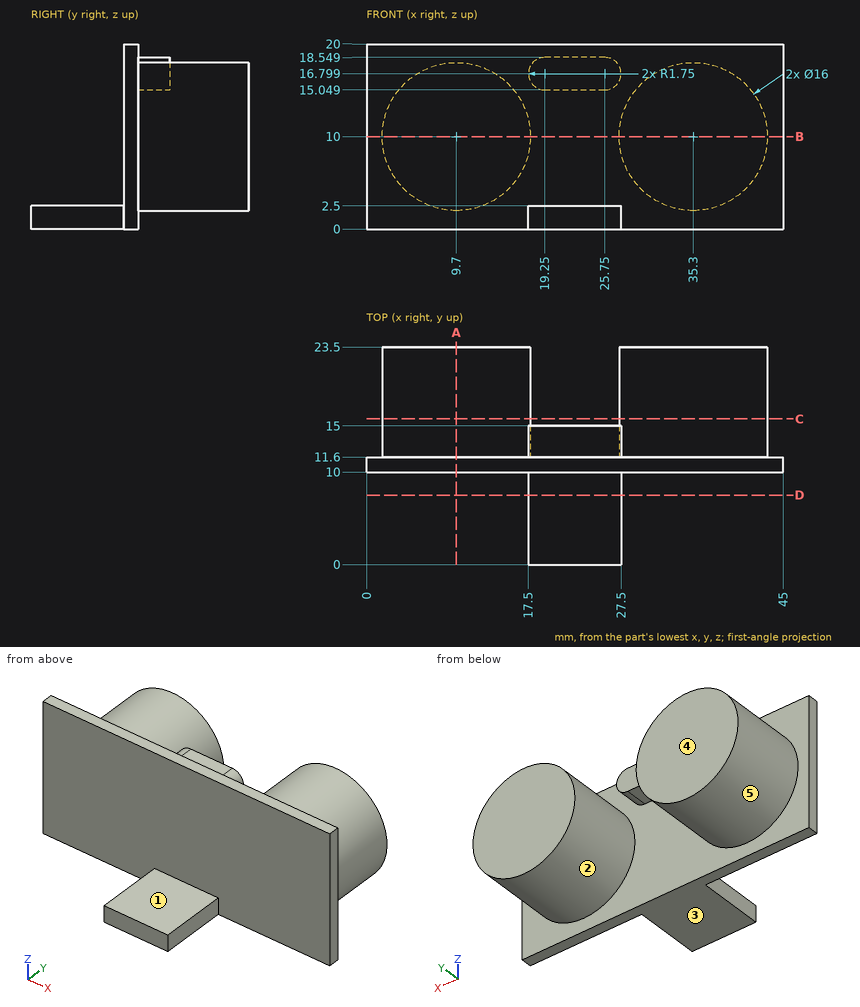
Can you work these out from the drawing? Everything is in mm from the part's minimum corner. A direction names the side the tool comes from. Round coordinates to 2 decimals unless told otherwise and drop trailing zeros. Loops run counter-clockwise (first coordinate to the right, second up) from the corner with the lowest first, then second, coordinate; pieces in that order, holes last. Notation, with made-up numbers: (-12, 2) - (-8, 2) arc R15 ccw to (-8, 25) - close; hole circle Ø1 at (-3, 57). An arc over 180 degrees is marked (long way). One line per question, with ' | ' between items. Start each with the question number.
Q1. I want a section at A-A (x = 9.7). Write out the boundary of the cut face in (y, z), then the cut area to 3 significant figures.
Q2. I want a section at B-B (z = 10). Write out the boundary of the cut face in (x, y).
Q3. I want a section at D-D (y = 7.5). Write out the boundary of the cut face in (x, z).
Q4. We'd pull the mould along X, two halves only. Please class the marked faces 4 and 5: +X half, -X half, draft (parallel to the pull), parting line (faces both ways), or undercut.
Q5. For the marked faces 1, 2 and 3, which set-ups out of +Z, -Z, +X, -X, +Y, -Y let a thin tool reach every point of the face, with its end or its side?
Q6. I want a section at C-C (y = 15.75). Write out the boundary of the cut face in (x, z), then the cut area to 3 significant figures.
Q7. Will these pins go through, and if not, where does the flat tip stop? pin 1 (8 mm diameter, centred on x = 29.5, y = 18.5, fed in from -Z) (1 decimal); pin 2 (1.7 mm diameter, centred on x = 23, y = 13.5, fed in from -Z); pin 3 (4 mm diameter, centred on x = 24, z = 17, fed in from +Y).
Q8. Please list where these lines run through material, in increasing order: line 1 (Y direction, x = 33.5, z = 4.25); line 2 (Z direction, x = 23, y = 3.25); line 3 (Y direction, x = 21.5, z = 1.5). Write a range as [from, to].
Response values:
1) outline: (10, 0) - (11.6, 0) - (11.6, 2) - (23.5, 2) - (23.5, 18) - (11.6, 18) - (11.6, 20) - (10, 20) - close | area: 222 mm²
2) outline: (0, 10) - (45, 10) - (45, 11.6) - (43.3, 11.6) - (43.3, 23.5) - (27.3, 23.5) - (27.3, 11.6) - (17.7, 11.6) - (17.7, 23.5) - (1.7, 23.5) - (1.7, 11.6) - (0, 11.6) - close
3) outline: (17.5, 0) - (27.5, 0) - (27.5, 2.5) - (17.5, 2.5) - close
4) face 4: draft | face 5: undercut
5) face 1: +Z, +X, -X, -Y | face 2: +Y | face 3: -Z, +X, -X, +Y, -Y
6) outline: circle Ø16 at (9.7, 10); circle Ø16 at (35.3, 10) | area: 402 mm²
7) pin 1: stops at z = 2.2 | pin 2: stops at z = 15.05 | pin 3: stops at y = 15
8) line 1: y = [10, 23.5] | line 2: z = [0, 2.5] | line 3: y = [0, 11.6]
